Input: part model. Units: mm. Frame: model coordinates. Face numbers are marked on the shaded views. A direction names the side the tool comes from. Give positions to 0.01 mm unless a question says otherwise; leave off trailing zeros. Order: outer loops, then holes, each group sorted by start corner. A loop starts at its lowest first (then second) coordinate and runs counter-clockwise, first axis right, second up. Notation, with made-up numbers: (18, -24) - (57, -24) arc R12 cw to (57, -15) - close; hole circle Ø9 at (17.25, -4). An arc over 180 degrees is marked (long way). Use a Markdown table: item, result.
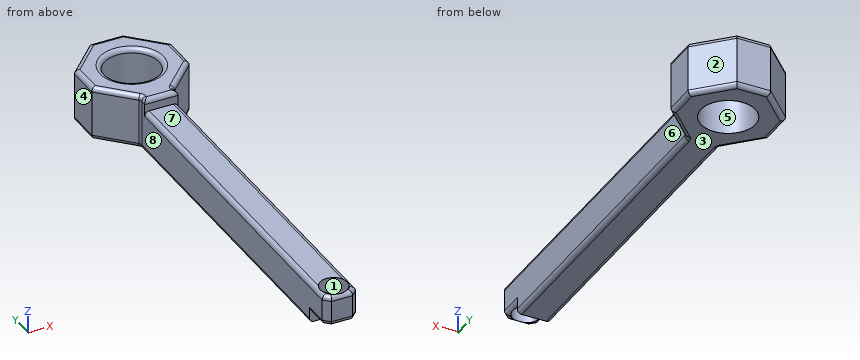
from build123d import *

# Parameters (mm, degrees)
SKETCH1_R               = 9
SKETCH1_R_2             = 4.5
BOSS_EXTRUDE1_DEPTH     = 18
CUT_EXTRUDE1_DEPTH      = 86.684353416
CUT_EXTRUDE1_DEPTH_BACK = 86.684353416
FILLET1_R               = 1.5


with BuildPart() as part:
    # Sketch1 → Boss-Extrude1 (new body)
    with BuildSketch(Plane.XY):
        Polygon((-7.557553962, -67.195132078), (-7.557553962, 48.266235791), (-18.143619364, 59.093986602), (-18.143619364, 70.115749241), (-7.557553962, 80.943500052), (3.442446038, 80.943500052), (14.02851144, 70.115749241), (14.02851144, 59.093986602), (3.442446038, 48.266235791), (3.442446038, -67.195132078), (1.442446038, -69.195132078), (-5.557553962, -69.195132078), align=None)
        with Locations((-2.057553962, 64.604867922)):
            Circle(SKETCH1_R, mode=Mode.SUBTRACT)
        with Locations((-2.057553962, -63.895132078)):
            Circle(SKETCH1_R_2, mode=Mode.SUBTRACT)
    extrude(amount=BOSS_EXTRUDE1_DEPTH)

    # Sketch2 → Cut-Extrude1 (cut, two sides: drawn at the far end of the back side and taken through both)
    with BuildSketch(Plane.ZY.offset(7.557553962).offset(-CUT_EXTRUDE1_DEPTH_BACK)):
        Polygon((3.920552613, -84.398483755), (3.920552613, -59.021038695), (-18.582585697, -59.021038695), (-18.582585697, -119.504750135), (35.581125662, -119.504750135), (35.581125662, 45.802779434), (13.920552613, 45.802779434), (13.920552613, -84.398483755), align=None)
    extrude(amount=CUT_EXTRUDE1_DEPTH + CUT_EXTRUDE1_DEPTH_BACK, mode=Mode.SUBTRACT)

    # Fillet1
    # the kernel refuses this fillet: 1.5 mm, written as the material it adds along each edge
    with BuildSketch(Plane(origin=(3.442446038, 48.266235791, 0), x_dir=(0, -1, 0), z_dir=(0, 0, 1))) as fillet1_piece_1:
        with BuildLine():
            CenterArc((FILLET1_R * 0.407617755976, FILLET1_R), FILLET1_R, 225.646637005, 44.353362995)
            Line((-FILLET1_R * 0.291463794008, FILLET1_R * 0.284958052649), (0, 0))
            Line((0, 0), (FILLET1_R * 0.407617755976, 0))
        make_face()
    extrude(amount=18)
    with BuildSketch(Plane(origin=(-7.557553962, 48.266235791, 0), x_dir=(0, -1, 0), z_dir=(0, 0, 1))) as fillet1_piece_2:
        with BuildLine():
            CenterArc((FILLET1_R * 0.407617755976, -FILLET1_R), FILLET1_R, 90, 44.353362995)
            Line((-FILLET1_R * 0.291463794008, -FILLET1_R * 0.284958052649), (0, 0))
            Line((0, 0), (FILLET1_R * 0.407617755976, 0))
        make_face()
    extrude(amount=18)
    # the kernel refuses this fillet: 1.5 mm, written as the material it takes off along each edge
    with BuildSketch(Plane(origin=(-18.143619364, 55.343986602, 0), x_dir=(1, 0, 0), z_dir=(0, 1, 0)), Plane(origin=(14.02851144, 73.865749241, 0), x_dir=(-1, 0, 0), z_dir=(0, -1, 0))) as fillet1_2_piece_1:
        with BuildLine():
            CenterArc((FILLET1_R, -FILLET1_R), FILLET1_R, 90, 90)
            Line((0, -FILLET1_R), (0, 0))
            Line((0, 0), (FILLET1_R, 0))
        make_face()
    extrude(amount=18.521762639, mode=Mode.SUBTRACT)
    with BuildSketch(Plane(origin=(-20.765175176, 67.434341939, 0), x_dir=(0.7150419473513874, -0.6990815499839313, 0), z_dir=(0.6990815499839312, 0.7150419473513874, 0)), Plane(origin=(0.820890226, 83.624907355, 0), x_dir=(-0.7150419473513874, -0.6990815499839313, 0), z_dir=(0.6990815499839312, -0.7150419473513874, 0))) as fillet1_2_piece_2:
        with BuildLine():
            CenterArc((FILLET1_R, -FILLET1_R), FILLET1_R, 90, 90)
            Line((0, -FILLET1_R), (0, 0))
            Line((0, 0), (FILLET1_R, 0))
        make_face()
    extrude(amount=22.642819035, mode=Mode.SUBTRACT)
    with BuildSketch(Plane(origin=(-11.307553962, 80.943500052, 0), x_dir=(0, -1, 0), z_dir=(1, 0, 0))) as fillet1_2_piece_3:
        with BuildLine():
            CenterArc((FILLET1_R, -FILLET1_R), FILLET1_R, 90, 90)
            Line((0, -FILLET1_R), (0, 0))
            Line((0, 0), (FILLET1_R, 0))
        make_face()
    extrude(amount=18.5, mode=Mode.SUBTRACT)
    with BuildSketch(Plane(origin=(16.650067253, 61.775393905, 0), x_dir=(-0.7150419473513876, 0.699081549983931, 0), z_dir=(-0.699081549983931, -0.7150419473513876, 0)), Plane(origin=(-7.984991041, 48.703431482, 0), x_dir=(0.7150419473513876, 0.699081549983931, 0), z_dir=(-0.699081549983931, 0.7150419473513876, 0))) as fillet1_2_piece_4:
        with BuildLine():
            CenterArc((FILLET1_R, -FILLET1_R), FILLET1_R, 90, 90)
            Line((0, -FILLET1_R), (0, 0))
            Line((0, 0), (FILLET1_R, 0))
        make_face()
    extrude(amount=18.281392401, mode=Mode.SUBTRACT)
    with BuildSketch(Plane(origin=(-7.557553962, -62.771038695, 0), x_dir=(0, 0, 1), z_dir=(0, 1, 0))) as fillet1_2_piece_5:
        with BuildLine():
            CenterArc((FILLET1_R, FILLET1_R), FILLET1_R, 180, 90)
            Line((0, FILLET1_R), (0, 0))
            Line((0, 0), (FILLET1_R, 0))
        make_face()
    extrude(amount=110.425847852, mode=Mode.SUBTRACT)
    with BuildSketch(Plane(origin=(16.650067253, 61.775393905, 18), x_dir=(-0.7150419473513876, 0.699081549983931, 0), z_dir=(-0.699081549983931, -0.7150419473513876, 0)), Plane(origin=(-7.984991041, 48.703431482, 18), x_dir=(0.7150419473513876, 0.699081549983931, 0), z_dir=(-0.699081549983931, 0.7150419473513876, 0))) as fillet1_2_piece_6:
        with BuildLine():
            CenterArc((FILLET1_R, FILLET1_R), FILLET1_R, 180, 90)
            Line((0, FILLET1_R), (0, 0))
            Line((0, 0), (FILLET1_R, 0))
        make_face()
    extrude(amount=18.281392401, mode=Mode.SUBTRACT)
    with BuildSketch(Plane(origin=(-2.057553962, 64.604867922, 18), x_dir=(1, 0, 0), z_dir=(0, -1, 0))) as fillet1_2_piece_7:
        with BuildLine():
            CenterArc((9 + FILLET1_R, -FILLET1_R), FILLET1_R, 90, 90)
            Line((9, -FILLET1_R), (9, 0))
            Line((9, 0), (9 + FILLET1_R, 0))
        make_face()
    revolve(axis=Axis((-2.057553962, 64.604867922, 18), (0, 0, 1)), mode=Mode.SUBTRACT)
    with BuildSketch(Plane(origin=(14.02851144, 73.865749241, 18), x_dir=(-1, 0, 0), z_dir=(0, -1, 0)), Plane(origin=(-18.143619364, 55.343986602, 18), x_dir=(1, 0, 0), z_dir=(0, 1, 0))) as fillet1_2_piece_8:
        with BuildLine():
            CenterArc((FILLET1_R, FILLET1_R), FILLET1_R, 180, 90)
            Line((0, FILLET1_R), (0, 0))
            Line((0, 0), (FILLET1_R, 0))
        make_face()
    extrude(amount=18.521762639, mode=Mode.SUBTRACT)
    with BuildSketch(Plane(origin=(0.820890226, 83.624907355, 18), x_dir=(-0.7150419473513874, -0.6990815499839313, 0), z_dir=(0.6990815499839312, -0.7150419473513874, 0)), Plane(origin=(-20.765175176, 67.434341939, 18), x_dir=(0.7150419473513874, -0.6990815499839313, 0), z_dir=(0.6990815499839312, 0.7150419473513874, 0))) as fillet1_2_piece_9:
        with BuildLine():
            CenterArc((FILLET1_R, FILLET1_R), FILLET1_R, 180, 90)
            Line((0, FILLET1_R), (0, 0))
            Line((0, 0), (FILLET1_R, 0))
        make_face()
    extrude(amount=22.642819035, mode=Mode.SUBTRACT)
    with BuildSketch(Plane(origin=(-11.307553962, 80.943500052, 18), x_dir=(0, -1, 0), z_dir=(1, 0, 0)), Plane(origin=(7.192446038, 45.802779434, 18), x_dir=(0, 1, 0), z_dir=(-1, 0, 0))) as fillet1_2_piece_10:
        with BuildLine():
            CenterArc((FILLET1_R, FILLET1_R), FILLET1_R, 180, 90)
            Line((0, FILLET1_R), (0, 0))
            Line((0, 0), (FILLET1_R, 0))
        make_face()
    extrude(amount=18.5, mode=Mode.SUBTRACT)
    with BuildSketch(Plane(origin=(3.442446038, 47.654809157, 0), x_dir=(-1, 0, 0), z_dir=(0, -1, 0))) as fillet1_2_piece_11:
        with BuildLine():
            CenterArc((FILLET1_R, -FILLET1_R), FILLET1_R, 90, 90)
            Line((0, -FILLET1_R), (0, 0))
            Line((0, 0), (FILLET1_R, 0))
        make_face()
    extrude(amount=110.425847852, mode=Mode.SUBTRACT)
    with BuildSketch(Plane(origin=(3.442446038, 47.654809157, 18), x_dir=(-1, 0, 0), z_dir=(0, -1, 0))) as fillet1_2_piece_12:
        with BuildLine():
            CenterArc((FILLET1_R, FILLET1_R), FILLET1_R, 180, 90)
            Line((0, FILLET1_R), (0, 0))
            Line((0, 0), (FILLET1_R, 0))
        make_face()
    extrude(amount=5.602029724, mode=Mode.SUBTRACT)
    with BuildSketch(Plane(origin=(-2.905903532, -71.846782508, 13.920552613), x_dir=(0.7071067811865479, 0.707106781186547, 0), z_dir=(-0.7071067811865471, 0.707106781186548, 0)), Plane(origin=(6.094096468, -64.543481649, 13.920552613), x_dir=(-0.7071067811865501, 0.7071067811865448, 0), z_dir=(-0.7071067811865448, -0.7071067811865502, 0)), Plane(origin=(-1.209204391, -71.846782508, 3.920552613), x_dir=(-0.7071067811865502, 0.7071067811865449, 0), z_dir=(0.7071067811865448, 0.7071067811865502, 0))) as fillet1_2_piece_13:
        with BuildLine():
            CenterArc((FILLET1_R, FILLET1_R), FILLET1_R, 180, 90)
            Line((0, FILLET1_R), (0, 0))
            Line((0, 0), (FILLET1_R, 0))
        make_face()
    extrude(amount=10.328427125, mode=Mode.SUBTRACT)
    with BuildSketch(Plane(origin=(-7.557553962, -70.945132078, 13.920552613), x_dir=(0, 0, -1), z_dir=(0, 1, 0))) as fillet1_2_piece_14:
        with BuildLine():
            CenterArc((FILLET1_R, -FILLET1_R), FILLET1_R, 90, 90)
            Line((0, -FILLET1_R), (0, 0))
            Line((0, 0), (FILLET1_R, 0))
        make_face()
    extrude(amount=116.747911512, mode=Mode.SUBTRACT)
    with BuildSketch(Plane(origin=(3.442446038, 45.802779434, 13.920552613), x_dir=(-1, 0, 0), z_dir=(0, -1, 0))) as fillet1_2_piece_15:
        with BuildLine():
            CenterArc((FILLET1_R, FILLET1_R), FILLET1_R, 180, 90)
            Line((0, FILLET1_R), (0, 0))
            Line((0, 0), (FILLET1_R, 0))
        make_face()
    extrude(amount=116.747911512, mode=Mode.SUBTRACT)
    with BuildSketch(Plane(origin=(5.192446038, -69.195132078, 13.920552613), x_dir=(0, 1, 0), z_dir=(-1, 0, 0)), Plane(origin=(-9.307553962, -69.195132078, 3.920552613), x_dir=(0, 1, 0), z_dir=(1, 0, 0))) as fillet1_2_piece_16:
        with BuildLine():
            CenterArc((FILLET1_R, FILLET1_R), FILLET1_R, 180, 90)
            Line((0, FILLET1_R), (0, 0))
            Line((0, 0), (FILLET1_R, 0))
        make_face()
    extrude(amount=14.5, mode=Mode.SUBTRACT)
    with BuildSketch(Plane(origin=(-7.557553962, -59.021038695, 3.920552613), x_dir=(0, 0, 1), z_dir=(0, -1, 0))) as fillet1_2_piece_17:
        with BuildLine():
            CenterArc((FILLET1_R, -FILLET1_R), FILLET1_R, 90, 90)
            Line((0, -FILLET1_R), (0, 0))
            Line((0, 0), (FILLET1_R, 0))
        make_face()
    extrude(amount=11.924093383, mode=Mode.SUBTRACT)
    with BuildSketch(Plane(origin=(-10.209204391, -64.543481649, 3.920552613), x_dir=(0, 0, 1), z_dir=(0.7071067811865471, -0.707106781186548, 0))) as fillet1_2_piece_18:
        with BuildLine():
            CenterArc((FILLET1_R, -FILLET1_R), FILLET1_R, 90, 90)
            Line((0, -FILLET1_R), (0, 0))
            Line((0, 0), (FILLET1_R, 0))
        make_face()
    extrude(amount=10.328427125, mode=Mode.SUBTRACT)
    with BuildSketch(Plane(origin=(3.442446038, -70.945132078, 3.920552613), x_dir=(-1, 0, 0), z_dir=(0, 1, 0))) as fillet1_2_piece_19:
        with BuildLine():
            CenterArc((FILLET1_R, FILLET1_R), FILLET1_R, 180, 90)
            Line((0, FILLET1_R), (0, 0))
            Line((0, 0), (FILLET1_R, 0))
        make_face()
    extrude(amount=11.924093383, mode=Mode.SUBTRACT)
    with BuildSketch(Plane(origin=(-7.557553962, 42.052779434, 18), x_dir=(0, 0, -1), z_dir=(0, 1, 0))) as fillet1_2_piece_20:
        with BuildLine():
            CenterArc((FILLET1_R, -FILLET1_R), FILLET1_R, 90, 90)
            Line((0, -FILLET1_R), (0, 0))
            Line((0, 0), (FILLET1_R, 0))
        make_face()
    extrude(amount=5.602029724, mode=Mode.SUBTRACT)
    with BuildSketch(Plane(origin=(-9.057553962, 47.654809157, 18), x_dir=(1, 0, 0), z_dir=(0, -1, 0))) as fillet1_2_piece_21:
        with BuildLine():
            CenterArc((1.5 + FILLET1_R, -FILLET1_R), FILLET1_R, 90, 90)
            Line((1.5 + FILLET1_R, 0), (1.5, 0))
            Line((1.5, 0), (1.5, -FILLET1_R))
        make_face()
    revolve(axis=Axis((-9.057553962, 47.654809157, 18), (0, 0, 1)), revolution_arc=44.353362995, mode=Mode.SUBTRACT)
    with BuildSketch(Plane(origin=(4.942446038, 47.654809157, 18), x_dir=(-1, 0, 0), z_dir=(0, -1, 0))) as fillet1_2_piece_22:
        with BuildLine():
            CenterArc((1.5 + FILLET1_R, FILLET1_R), FILLET1_R, 180, 90)
            Line((1.5, FILLET1_R), (1.5, 0))
            Line((1.5, 0), (1.5 + FILLET1_R, 0))
        make_face()
    revolve(axis=Axis((4.942446038, 47.654809157, 18), (0, 0, -1)), revolution_arc=44.353362995, mode=Mode.SUBTRACT)
    with BuildSketch(Plane(origin=(4.942446038, 47.654809157, 0), x_dir=(-1, 0, 0), z_dir=(0, -1, 0))) as fillet1_2_piece_23:
        with BuildLine():
            CenterArc((1.5 + FILLET1_R, -FILLET1_R), FILLET1_R, 90, 90)
            Line((1.5, -FILLET1_R), (1.5, 0))
            Line((1.5, 0), (1.5 + FILLET1_R, 0))
        make_face()
    revolve(axis=Axis((4.942446038, 47.654809157, 0), (0, 0, -1)), revolution_arc=44.353362995, mode=Mode.SUBTRACT)
    with BuildSketch(Plane(origin=(-9.057553962, 47.654809157, 0), x_dir=(1, 0, 0), z_dir=(0, -1, 0))) as fillet1_2_piece_24:
        with BuildLine():
            CenterArc((1.5 + FILLET1_R, FILLET1_R), FILLET1_R, 180, 90)
            Line((1.5, FILLET1_R), (1.5, 0))
            Line((1.5, 0), (1.5 + FILLET1_R, 0))
        make_face()
    revolve(axis=Axis((-9.057553962, 47.654809157, 0), (0, 0, 1)), revolution_arc=44.353362995, mode=Mode.SUBTRACT)


solid = part.part
1. Mould query, pull axis X, two halves, no side actions, for the marked faces 1, 2 and 3. Classes: pulls with the +X half, pulls with the -X half, needs draft (parallel to the pull), parting line crosses it, or undercut.
Response:
| item | result |
|---|---|
| face 1 | undercut |
| face 2 | pulls with the +X half |
| face 3 | needs draft |
2. Section query B-B (z = 8). Return loops of the section in (x, y) (1 decimal), then the cut area to 3 significant figures.
Response:
| item | result |
|---|---|
| outline | (-18.1, 59.1) - (-8, 48.7) arc R1.5 cw to (-7.6, 47.7) - (-7.6, -67.2) - (-5.6, -69.2) - (1.4, -69.2) - (3.4, -67.2) - (3.4, 47.7) arc R1.5 cw to (3.9, 48.7) - (14, 59.1) - (14, 70.1) - (3.4, 80.9) - (-7.6, 80.9) - (-18.1, 70.1) - close; hole circle Ø18 at (-2.1, 64.6); hole circle Ø9 at (-2.1, -63.9) |
| area | 1,790 mm^2 |
3. Section query C-C (x = -1). State how many separate pieces and enclosed holes the cut face has, then the cut area to 3 significant figures.
Response:
| item | result |
|---|---|
| separate pieces | 3 |
| enclosed holes | 0 |
| area | 1,780 mm^2 |
4. Set-up query: the marked faces 4, 5, 6, 7 and 8. Return all of +Z, -Z, +X, -X, +Y, -Y with unobstructed straight access to the full face (end or side cutting, diameter ignored); none if empty.
Response:
| item | result |
|---|---|
| face 4 | +Z, -Z, -X, +Y, -Y |
| face 5 | +Z, -Z |
| face 6 | +Z, -Z, +X, -Y |
| face 7 | +Z, +X, -X, -Y |
| face 8 | +Z, -Z, -X, -Y |
5. Material intervals for line 1 along Y through (x, z) = (2, 5); line 2 along Y through (x, z) = (-6, 8); line 3 along X through (y, z) = (58, 8.75), sorted ascending.
Response:
| item | result |
|---|---|
| line 1 | y = -68.55 to -65.84, -61.95 to 56.57, 72.64 to 80.94 |
| line 2 | y = -68.75 to -66.06, -61.73 to 56.51, 72.7 to 80.94 |
| line 3 | x = -17.07 to -8.17, 4.06 to 12.96 |
6. Pin query (flat end, axial travel): pin 1 (1 mm diameter, centred on y = -28.5, z = 14.5, fed in from -X); pin 2 (2.5 mm diameter, centred on x = -3.5, y = -60, fed in from -Z); pin 3 (5 mm diameter, centred on y = -38, z = 15, fed in from -X); pin 4 (1.5 mm diameter, centred on x = 8, z = 7.5, fed in from -Y). Return the tip coordinate at first contact, or that it passes through.
Response:
| item | result |
|---|---|
| pin 1 | passes through |
| pin 2 | stops at z = 0 |
| pin 3 | stops at x = -7.56 |
| pin 4 | stops at y = 52.16 |
7. Section query A-A (y = -21). Return loops of the section in (x, z).
Response:
| item | result |
|---|---|
| outline | (-7.56, 1.5) arc R1.5 ccw to (-6.06, 0) - (1.94, 0) arc R1.5 ccw to (3.44, 1.5) - (3.44, 12.42) arc R1.5 ccw to (1.94, 13.92) - (-6.06, 13.92) arc R1.5 ccw to (-7.56, 12.42) - close |
